Source: CAD feature listing. Evaluate the final solid. Frame: model axes, mm. Give positions to 0.01 mm unless a question says otherwise; leave off trailing zeros. Loops run counter-clockwise (first coordinate to the right, second up) from the corner with the lowest first, then second, coordinate; pieces in that order, holes last. Notation, with made-up numbers: M 53,-11 L 75,-11 A9 ccw 75,0 Z; hole C 19,52 d2. An arc over 180 degrees is marked long. Put each result on its own line as item: value.
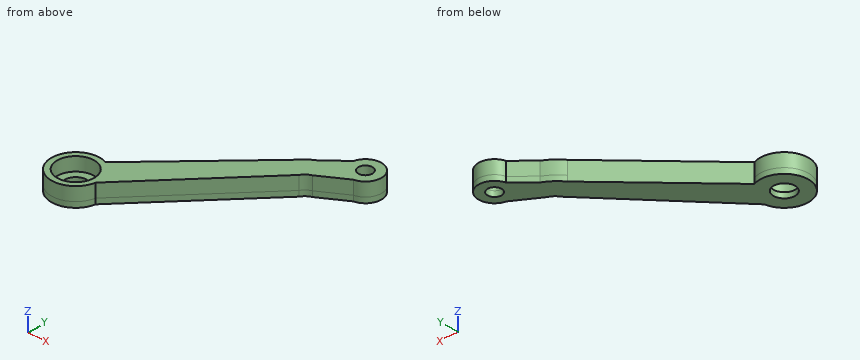
from build123d import *

# Parameters (mm, degrees)
SKETCH1_R           = 2.6
SKETCH1_R_2         = 6.9
BOSS_EXTRUDE1_DEPTH = 5
BOSS_EXTRUDE2_START = 2
SKETCH2_R           = 4
SKETCH2_R_2         = 2.6
BOSS_EXTRUDE2_DEPTH = 2
SCALE1_SCALE        = 1.5


with BuildPart() as part:
    # Sketch1 → Boss-Extrude1 (new body)
    with BuildSketch(Plane.XY):
        with BuildLine():
            Line((-116.116459466, -73.116163472), (-77.780395614, -32.221656848))
            ThreePointArc((-77.780395614, -32.221656848), (-76.528201342, -30.740668075), (-74.833515464, -29.797610273))
            Line((-74.833515464, -29.797610273), (-65.058269204, -23.896184603))
            ThreePointArc((-65.058269204, -23.896184603), (-61.52405595, -14.086356432), (-71.687164611, -16.417582375))
            Line((-71.687164611, -16.417582375), (-78.635941465, -22.763122171))
            ThreePointArc((-78.635941465, -22.763122171), (-81.861894444, -24.820779517), (-84.529701766, -27.563684997))
            Line((-84.529701766, -27.563684997), (-121.430579381, -63.327828505))
            ThreePointArc((-121.430579381, -63.327828505), (-132.896560675, -75.889442497), (-116.116459466, -73.116163472))
        make_face()
        with Locations((-65.969197132, -18.026447785)):
            Circle(SKETCH1_R, mode=Mode.SUBTRACT)
        with Locations((-124.987033061, -71.595333402)):
            Circle(SKETCH1_R_2, mode=Mode.SUBTRACT)
    extrude(amount=BOSS_EXTRUDE1_DEPTH)

    # Sketch2 → Boss-Extrude2 (add)
    with BuildSketch(Plane(origin=(0, 0, 0), x_dir=(-1, 0, 0), z_dir=(0, 0, -1)).offset(BOSS_EXTRUDE2_START)):
        with BuildLine():
            Line((121.430579381, -63.327828505), (84.529701766, -27.563684997))
            ThreePointArc((84.529701766, -27.563684997), (81.861894444, -24.820779517), (78.635941465, -22.763122171))
            Line((78.635941465, -22.763122171), (71.687164611, -16.417582375))
            ThreePointArc((71.687164611, -16.417582375), (61.52405595, -14.086356432), (65.058269204, -23.896184603))
            Line((65.058269204, -23.896184603), (74.833515464, -29.797610273))
            ThreePointArc((74.833515464, -29.797610273), (76.528201342, -30.740668075), (77.780395614, -32.221656848))
            Line((77.780395614, -32.221656848), (116.116459466, -73.116163472))
            ThreePointArc((116.116459466, -73.116163472), (132.896560675, -75.889442497), (121.430579381, -63.327828505))
        make_face()
        with Locations((124.987033061, -71.595333402)):
            Circle(SKETCH2_R, mode=Mode.SUBTRACT)
        with Locations((65.969197132, -18.026447785)):
            Circle(SKETCH2_R_2, mode=Mode.SUBTRACT)
    extrude(amount=-BOSS_EXTRUDE2_DEPTH)


with BuildPart() as part_1:
    # Scale1: scaled about (-96.971512975, -46.1293356, 1.414619299)
    add(part.part.scale(SCALE1_SCALE).moved(Location((48.485756487, 23.0646678, -0.707309649))))


solid = part_1.part
1. Section query C-C (z = -2.25). Output: boundary loops of the cut face in (x, y) (3 decimals), plus the area to 3 significant figures.
Found:
outline: M -133.66,-71.927 A13.5 ccw long -125.689,-86.61 L -68.185,-25.268 A8.1 cw -63.765,-21.632 L -49.102,-12.78 A8.91 ccw long -59.045,-1.562 L -69.468,-11.08 A24.849 ccw -78.309,-18.281 Z; hole C -138.995,-84.328 d12; hole C -50.468,-3.975 d7.8
area: 2,030 mm^2
2. Contact query for flat-ended pins moving along their axis: P1, Ø1.5, axis at x = -81.5, z = 5, coming from the -Y side; P2, Ø1.5, axis at y = -39, z = 4.5, coming from the +X side. Output: stop coordinate, or through.
Found:
P1: y = -40.27
P2: x = -80.35
3. Section query D-D (z = 4.75). Output: boundary loops of the cut face in (x, y) (3 decimals), plus the area to 3 significant figures.
Found:
outline: M -133.66,-71.927 A13.5 ccw long -125.689,-86.61 L -68.185,-25.268 A8.1 cw -63.765,-21.632 L -49.102,-12.78 A8.91 ccw long -59.045,-1.562 L -69.468,-11.08 A24.849 ccw -78.309,-18.281 Z; hole C -138.995,-84.328 d20.7; hole C -50.468,-3.975 d7.8
area: 1,810 mm^2
4. Section query B-B (y = -80.5). Output: boundary loops of the cut face in (x, z), plus the area to 3 significant figures.
Found:
outline: M -151.94,-3.71 L -143.61,-3.71 L -143.61,-0.71 L -148.61,-0.71 L -148.61,6.79 L -151.94,6.79 Z; M -134.37,-3.71 L -119.96,-3.71 L -119.96,6.79 L -129.38,6.79 L -129.38,-0.71 L -134.37,-0.71 Z
area: 164 mm^2
5. Material intervals for line 1 (Y direction, x = -52.5, z = -1); line 2 (Y direction, x = -146.5, z = 0.75); line 3 (X direction, y = -93, z = -0.5), sorted ascending. Write a range as from..to.
Found:
line 1: -14.83..-7.3, -0.65..4.7
line 2: -95.55..-91.46, -77.2..-73.11
line 3: -149.34..-144.64, -133.34..-128.65
6. Section query A-A (x = -135.5). Output: boundary loops of the cut face in (y, z), plus the area to 3 significant figures.
Found:
outline: M -97.37,-3.71 L -89.21,-3.71 L -89.21,-0.71 L -94.07,-0.71 L -94.07,6.79 L -97.37,6.79 Z; M -79.45,-3.71 L -71.29,-3.71 L -71.29,6.79 L -74.59,6.79 L -74.59,-0.71 L -79.45,-0.71 Z
area: 98.4 mm^2
